Design review of the part built by this model. Coordinates are the model's own, in mm. Give positions to 0.01 mm unless a question says otherwise; leave off trailing zeros. Order: outer loops, then holes, each group sorted by start corner. A loop starts at its lowest first (then second) coordinate and runs counter-clockwise, first axis right, second up. Notation, with made-up numbers: (-3.5, 61) -> (1.5, 61) arc R20 cw to (1.5, 85) -> close; hole circle Ø1 at (4.5, 62.25). An arc over 180 degrees is marked (long way). Return JSON: item names as keys, results as strings.
```python
from build123d import *

# Parameters (mm, degrees)
SKETCH1_W               = 539
SKETCH1_H               = 299
BOSS_EXTRUDE1_DEPTH     = 14
SKETCH15_W              = 70
SKETCH15_H              = 20
CUT_EXTRUDE8_DEPTH      = 309.506888092
SKETCH2_W               = 30
SKETCH2_H               = 51
CUT_EXTRUDE1_DEPTH      = 309.506888092
SKETCH16_W              = 200
SKETCH16_H              = 60
CUT_EXTRUDE9_DEPTH      = 10
SKETCH17_R              = 10.5
CUT_EXTRUDE10_DEPTH     = 15
SKETCH18_R              = 10.5
CUT_EXTRUDE11_DEPTH     = 10
BOSS_EXTRUDE2_DEPTH     = 60
MIRROR4_COPY_1_SKETCH_R = 10.5
MIRROR4_COPY_1_DEPTH    = 10
M6_CLEARANCE_HOLE1_D    = 6.6
MIRROR7_COPY_1_D        = 6.6
SKETCH23_W              = 11
SKETCH23_H              = 104.5
CUT_EXTRUDE12_DEPTH     = 1.5
SKETCH24_W              = 20
SKETCH24_H              = 30
CUT_EXTRUDE13_DEPTH     = 8


with BuildPart() as part:
    # Sketch1 → Boss-Extrude1 (new body)
    with BuildSketch(Plane(origin=(0, 0, 0), x_dir=(1, 0, 0), z_dir=(0, 1, 0))):
        Rectangle(SKETCH1_W, SKETCH1_H)
    extrude(amount=-BOSS_EXTRUDE1_DEPTH)

    # Sketch15 → Cut-Extrude8 (cut, through all)
    with BuildSketch(Plane(origin=(0, 0, 0), x_dir=(1, 0, 0), z_dir=(0, 1, 0))):
        Polygon((269.5, 149.5), (199.5, 149.5), (199.5, 129.5), (249.5, 129.5), (249.5, 91.5), (269.5, 91.5), align=None)
        with Locations((234.5, -139.5)):
            Rectangle(SKETCH15_W, SKETCH15_H)
    extrude(amount=-CUT_EXTRUDE8_DEPTH, mode=Mode.SUBTRACT)

    # Sketch2 → Cut-Extrude1 (cut, through all)
    with BuildSketch(Plane(origin=(0, 0, 0), x_dir=(1, 0, 0), z_dir=(0, 1, 0))):
        with Locations((-254.5, 0)):
            Rectangle(SKETCH2_W, SKETCH2_H)
    cut_extrude1 = extrude(amount=-CUT_EXTRUDE1_DEPTH, mode=Mode.SUBTRACT)

    # Mirror1: Cut-Extrude1 across plane
    add(cut_extrude1.mirror(Plane(origin=(0, 0, 0), x_dir=(0, 0, 1), z_dir=(1, 0, 0))), mode=Mode.SUBTRACT)

    # Sketch16 → Cut-Extrude9 (cut)
    with BuildSketch(Plane(origin=(0, 0, 0), x_dir=(1, 0, 0), z_dir=(0, 1, 0))):
        Rectangle(SKETCH16_W, SKETCH16_H)
    extrude(amount=-CUT_EXTRUDE9_DEPTH, mode=Mode.SUBTRACT)

    # Sketch17 → Cut-Extrude10 (cut)
    with BuildSketch(Plane.XY.offset(-30)):
        with Locations((0, 1.5)):
            Circle(SKETCH17_R)
    cut_extrude10 = extrude(amount=-CUT_EXTRUDE10_DEPTH, mode=Mode.SUBTRACT)

    # Sketch18 → Cut-Extrude11 (cut)
    with BuildSketch(Plane.XY.offset(-30)):
        with Locations((-39.971865105, 1.5)):
            Circle(SKETCH18_R)
        with Locations((-79.971865105, 1.5)):
            Circle(SKETCH18_R)
    cut_extrude11 = extrude(amount=-CUT_EXTRUDE11_DEPTH, mode=Mode.SUBTRACT)

    # Sketch19 → Boss-Extrude2 (add)
    with BuildSketch(Plane.XY.offset(-30)):
        with BuildLine():
            Line((-9.5, -10), (-30.5, -10))
            ThreePointArc((-30.5, -10), (-20, 0.5), (-9.5, -10))
        make_face()
        with BuildLine():
            Line((-89.5, -10), (-100, -10))
            Line((-100, -10), (-100, 0))
            Line((-100, 0), (-96.798437881, 0))
            ThreePointArc((-96.798437881, 0), (-91.518655701, -3.809943548), (-89.5, -10))
        make_face()
        with BuildLine():
            Line((-49.5, -10), (-70.5, -10))
            ThreePointArc((-70.5, -10), (-60, 0.5), (-49.5, -10))
        make_face()
    boss_extrude2 = extrude(amount=BOSS_EXTRUDE2_DEPTH)

    # Mirror2: Boss-Extrude2 across plane
    add(boss_extrude2.mirror(Plane(origin=(0, 0, 0), x_dir=(0, 0, 1), z_dir=(1, 0, 0))))

    # Mirror3: Cut-Extrude11 across plane
    add(cut_extrude11.mirror(Plane(origin=(0, 0, 0), x_dir=(0, 0, 1), z_dir=(1, 0, 0))), mode=Mode.SUBTRACT)

    # Mirror4: Cut-Extrude10, Cut-Extrude11 across plane
    add(cut_extrude10.mirror(Plane.XY), mode=Mode.SUBTRACT)
    add(cut_extrude11.mirror(Plane.XY), mode=Mode.SUBTRACT)

    # Mirror4 copy 1 sketch → Mirror4 copy 1 (cut)
    with BuildSketch(Plane(origin=(0, 0, 30), x_dir=(-1, 0, 0), z_dir=(0, 0, -1))):
        with Locations((-39.971865105, 1.5)):
            Circle(MIRROR4_COPY_1_SKETCH_R)
        with Locations((-79.971865105, 1.5)):
            Circle(MIRROR4_COPY_1_SKETCH_R)
    extrude(amount=-MIRROR4_COPY_1_DEPTH, mode=Mode.SUBTRACT)

    # M6 Clearance Hole1 (through all)
    with Locations(Plane(origin=(-257.5, 0, 45), x_dir=(0, 0, 1), z_dir=(0, 1, 0))):
        with Locations((0, 0), (-18.019432511, 47.1), (-8.008018456, 94.2), (2.003395598, 141.3), (15, 188.4), (20, 235.5)):
            m6_clearance_hole1 = Hole(M6_CLEARANCE_HOLE1_D / 2)

    # Mirror6: M6 Clearance Hole1 across plane
    add(m6_clearance_hole1.mirror(Plane(origin=(0, 0, 0), x_dir=(0, 0, 1), z_dir=(1, 0, 0))), mode=Mode.SUBTRACT)

    # Mirror7: M6 Clearance Hole1 across plane
    add(m6_clearance_hole1.mirror(Plane.XY), mode=Mode.SUBTRACT)

    # Mirror7 copy 1 (through all)
    with Locations(Plane(origin=(257.5, 0, -45), x_dir=(0, 0, -1), z_dir=(0, 1, 0))):
        with Locations((0, 0), (-18.019432511, 47.1), (-8.008018456, 94.2), (2.003395598, 141.3), (15, 188.4), (20, 235.5)):
            Hole(MIRROR7_COPY_1_D / 2)

    # Sketch23 → Cut-Extrude12 (cut)
    with BuildSketch(Plane(origin=(0, 0, 0), x_dir=(1, 0, 0), z_dir=(0, 1, 0))):
        with Locations((0, 97.25)):
            Rectangle(SKETCH23_W, SKETCH23_H)
    cut_extrude12 = extrude(amount=-CUT_EXTRUDE12_DEPTH, mode=Mode.SUBTRACT)

    # Sketch24 → Cut-Extrude13 (cut)
    with BuildSketch(Plane(origin=(0, 0, 0), x_dir=(1, 0, 0), z_dir=(0, 1, 0))):
        with Locations((0, 149.5)):
            Rectangle(SKETCH24_W, SKETCH24_H)
    cut_extrude13 = extrude(amount=-CUT_EXTRUDE13_DEPTH, mode=Mode.SUBTRACT)

    # Mirror8: Cut-Extrude12, Cut-Extrude13 across plane
    add(cut_extrude12.mirror(Plane.XY), mode=Mode.SUBTRACT)
    add(cut_extrude13.mirror(Plane.XY), mode=Mode.SUBTRACT)


solid = part.part
```
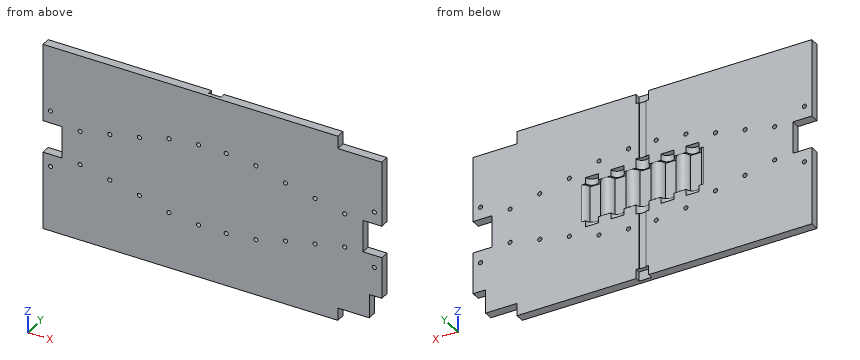
Item 1: Add section D-D (z = 10.5). Give the boundary of the cut face in (x, y).
Result set:
{"outline": "(-239.5, -14) -> (239.5, -14) -> (239.5, 0) -> (96.8, 0) arc R10.5 ccw to (89.5, -10) -> (70.5, -10) arc R10.5 ccw to (49.5, -10) -> (30.5, -10) arc R10.5 ccw to (9.5, -10) -> (-9.5, -10) arc R10.5 ccw to (-30.5, -10) -> (-49.5, -10) arc R10.5 ccw to (-70.5, -10) -> (-89.5, -10) arc R10.5 ccw to (-96.8, 0) -> (-239.5, 0) -> close"}
Item 2: Add section C-C (y = -5.25). Give the number of separate pieces and of enclosed holes in the cut face, plus the area to 3 significant figures.
Result set:
{"separate pieces": "1", "enclosed holes": "29", "area": "145,000 mm^2"}
Item 3: Add section A-A (z = -117.5). Give the boundary of the cut face in (x, y), plus the area to 3 significant figures.
Result set:
{"outline": "(-269.5, -14) -> (249.5, -14) -> (249.5, 0) -> (5.5, 0) -> (5.5, -1.5) -> (-5.5, -1.5) -> (-5.5, 0) -> (-269.5, 0) -> close", "area": "7,250 mm^2"}
Item 4: Add section B-B (x = 79.5). Give the boundary of the cut face in (y, z).
Result set:
{"outline": "(-14, -149.5) -> (0, -149.5) -> (0, -40) -> (-8.99, -40) -> (-8.99, -30) -> (-10, -30) -> (-10, 30) -> (-8.99, 30) -> (-8.99, 40) -> (0, 40) -> (0, 149.5) -> (-14, 149.5) -> close"}
Item 5: For pin 1 (4.5 mm diameter, centred on x = 3, z = -143, fed in from +Y); pin 2 (6 mm diameter, centred on x = 63, z = -93, fed in from +Y); pin 3 (8.5 mm diameter, centred on x = -116.2, z = 47, fed in from -Y); pin 4 (9.5 mm diameter, centred on x = -79, z = 1.5, fed in from +Y), all flat-tipped, find the tip position at first contact; note any pin that passes through.
Result set:
{"pin 1": "stops at y = -8", "pin 2": "stops at y = 0", "pin 3": "stops at y = -14", "pin 4": "stops at y = -10"}
Item 6: Wall thickness on L1, parallel to Z at x = 116.2, y = -5.5; L2, parallel to Z at x = -210.4, y = -4; L3, parallel to X at y = -3.25, z = -60: over which ranges is each line inside the solid? List them lowest first. Write a range as [from, to].
Result set:
{"L1": "z = [-149.5, -50.3], [-43.7, 43.7], [50.3, 149.5]", "L2": "z = [-149.5, -30.28], [-23.68, 23.68], [30.28, 149.5]", "L3": "x = [-269.5, -72.4], [-65.8, 65.8], [72.4, 269.5]"}
